```python
from build123d import *

# Parameters (mm, degrees)
TOP_PLATE_R             = 1
TOP_PLATE_R_2           = 2
TOP_PLATE_W             = 16.5
TOP_PLATE_H             = 8.5
TOP_PLATE_W_2           = 6
TOP_PLATE_H_2           = 18
TOP_PLATE_W_3           = 14
TOP_PLATE_H_3           = 12
TOP_PLATE_EXTRUDE_DEPTH = 2


with BuildPart() as part:
    # Top Plate → Top Plate Extrude (new body)
    with BuildSketch(Plane(origin=(0, 0, 0), x_dir=(1, 0, 0), z_dir=(0, 1, 0))):
        with BuildLine():
            Line((-38, 17.25), (-42.5, 17.25))
            Line((-42.5, 17.25), (-42.5, 14.926611549))
            Line((-42.5, 14.926611549), (-48, 14.926611549))
            Line((-48, 14.926611549), (-48, 10))
            Line((-48, 10), (-46.8, 10))
            ThreePointArc((-46.8, 10), (-46.587867966, 9.912132034), (-46.5, 9.7))
            Line((-46.5, 9.7), (-46.5, -9.7))
            ThreePointArc((-46.5, -9.7), (-46.587867966, -9.912132034), (-46.8, -10))
            Line((-46.8, -10), (-48, -10))
            Line((-48, -10), (-48, -14.926611549))
            Line((-48, -14.926611549), (-42.5, -14.926611549))
            Line((-42.5, -14.926611549), (-42.5, -17.25))
            Line((-42.5, -17.25), (-38, -17.25))
            Line((-38, -17.25), (-38, -14.926611549))
            Line((-38, -14.926611549), (-18, -14.926611549))
            Line((-18, -14.926611549), (-18, -17.25))
            Line((-18, -17.25), (-14, -17.25))
            Line((-14, -17.25), (-14, -14.926611549))
            Line((-14, -14.926611549), (6, -14.926611549))
            Line((6, -14.926611549), (6, -17.25))
            Line((6, -17.25), (10, -17.25))
            Line((10, -17.25), (10, -14.926611549))
            Line((10, -14.926611549), (34, -14.926611549))
            Line((34, -14.926611549), (34, -17.25))
            Line((34, -17.25), (47, -17.25))
            ThreePointArc((47, -17.25), (47.707106781, -16.957106781), (48, -16.25))
            Line((48, -16.25), (48, 16.25))
            ThreePointArc((48, 16.25), (47.707106781, 16.957106781), (47, 17.25))
            Line((47, 17.25), (34, 17.25))
            Line((34, 17.25), (34, 14.926611549))
            Line((34, 14.926611549), (10, 14.926611549))
            Line((10, 14.926611549), (10, 17.25))
            Line((10, 17.25), (6, 17.25))
            Line((6, 17.25), (6, 14.926611549))
            Line((6, 14.926611549), (-14, 14.926611549))
            Line((-14, 14.926611549), (-14, 17.25))
            Line((-14, 17.25), (-18, 17.25))
            Line((-18, 17.25), (-18, 14.926611549))
            Line((-18, 14.926611549), (-38, 14.926611549))
            Line((-38, 14.926611549), (-38, 17.25))
        make_face()
        with Locations(Location((-45.5, -11.5, 0), (0, 0, 270))):
            Circle(TOP_PLATE_R, mode=Mode.SUBTRACT)
        with Locations(Location((-41, -11.5, 0), (0, 0, 270))):
            Circle(TOP_PLATE_R, mode=Mode.SUBTRACT)
        with BuildLine():
            Line((-25, -10.5), (-13.5, -10.5))
            ThreePointArc((-13.5, -10.5), (-12.5, -11.5), (-13.5, -12.5))
            Line((-13.5, -12.5), (-25, -12.5))
            ThreePointArc((-25, -12.5), (-26, -11.5), (-25, -10.5))
        make_face(mode=Mode.SUBTRACT)
        with Locations(Location((44, -13.25, 0), (0, 0, 270))):
            Circle(TOP_PLATE_R_2, mode=Mode.SUBTRACT)
        with Locations((21.75, -6.75)):
            Rectangle(TOP_PLATE_W, TOP_PLATE_H, mode=Mode.SUBTRACT)
        with Locations((36, -0.25)):
            Rectangle(TOP_PLATE_W_2, TOP_PLATE_H_2, mode=Mode.SUBTRACT)
        with Locations((-31.5, 0)):
            Rectangle(TOP_PLATE_W_3, TOP_PLATE_H_3, mode=Mode.SUBTRACT)
        with Locations((-8.098292563, 0)):
            Rectangle(TOP_PLATE_W_3, TOP_PLATE_H_3, mode=Mode.SUBTRACT)
        with Locations(Location((-45.5, 11.5, 0), (0, 0, 270))):
            Circle(TOP_PLATE_R, mode=Mode.SUBTRACT)
        with Locations(Location((-41, 11.5, 0), (0, 0, 270))):
            Circle(TOP_PLATE_R, mode=Mode.SUBTRACT)
        with BuildLine():
            ThreePointArc((-13.5, 12.5), (-12.5, 11.5), (-13.5, 10.5))
            Line((-13.5, 10.5), (-25, 10.5))
            ThreePointArc((-25, 10.5), (-26, 11.5), (-25, 12.5))
            Line((-25, 12.5), (-13.5, 12.5))
        make_face(mode=Mode.SUBTRACT)
        Polygon((4.9, 9.249999917), (10.4, 9.249999917), (10.4, -8.75), (4.901707437, -8.750000002), align=None, mode=Mode.SUBTRACT)
        with Locations((21.75, 6.75)):
            Rectangle(TOP_PLATE_W, TOP_PLATE_H, mode=Mode.SUBTRACT)
        with BuildLine():
            ThreePointArc((42, 7.886262649), (43.5, 9.386262649), (45, 7.886262649))
            Line((45, 7.886262649), (45, -2.113737351))
            ThreePointArc((45, -2.113737351), (43.5, -3.613737351), (42, -2.113737351))
            Line((42, -2.113737351), (42, 7.886262649))
        make_face(mode=Mode.SUBTRACT)
        with Locations(Location((44, 12.75, 0), (0, 0, 270))):
            Circle(TOP_PLATE_R_2, mode=Mode.SUBTRACT)
    extrude(amount=TOP_PLATE_EXTRUDE_DEPTH)


solid = part.part
```
Verification items for the finished model (mm, model axes). A direction names the side the tool comes from. Round coordinates to 2 decimals unless told otherwise and drop trailing zeros. Order: outer loops, then holes, each group sorted by start corner. A loop starts at its lowest first (then second) coordinate and runs counter-clockwise, first axis right, second up. Notation, with made-up numbers: (77.5, 74) -> (106.5, 74) arc R6 ccw to (106.5, 82) -> close; hole circle Ø1 at (41, 33). An arc over 180 degrees is marked (long way). Put each result on its own line as item: value. Start each with the question number.
(1) Section check B-B (z = -1.5). Enter the section's corners in (x, y).
(2) Draft check along Z on faces 4 (the face through (-16, 1, -17.25)), 5 (the face through (43.467, 0.986, -9.386)), 6 (the face through (-40, 1, 17.25)). Enter one of: +Z half, -Z half, draft (parallel to the pull), parting line (faces both ways), or undercut.
(3) Tool access check on faces 1 (the face through (-18, 1, 16)), 2 (the face through (-4, 1, -14.927)), 3 (the face through (33, 1, 0)). Record the directions out of +Z, -Z, +X, -X, +Y, -Y that give a thin tool (end or side, any length) a straight path to the whole face; none if there is none.
(4) Section check C-C (x = 22). Enter the section's corners in (y, z), then the cut area to 3 significant figures.
(5) Section check A-A (x = 36). Enter the section's corners in (y, z), then the cut area to 3 significant figures.
(6) Material ranges on line 1 along X through (y, z) = (1.65, 4.5); line 2 along X through (y, z) = (0.2, -16); line 3 along X through (y, z) = (0.8, -7.5), recorded low to high.
(7) Depth check by flat-ended pin: pin 1 Ø2 at (x, z) = (-37, -4) entering from -Y; pin 2 Ø0.6 at (x, y) = (-4, 1.5) entering from +Z; pin 3 Ø0.6 at (x, y) = (-6.5, 1) entering from -Z. Enter the tip coordinate at first touch or a pass-through.
(8) Section check D-D (y = 1.1). State how many separate pieces and enclosed holes the cut face has, then the cut area to 3 significant figures.
Completed:
1. outline: (-46.5, 0) -> (-38.5, 0) -> (-38.5, 2) -> (-46.5, 2) -> close; (-24.5, 0) -> (-15.1, 0) -> (-15.1, 2) -> (-24.5, 2) -> close; (-1.1, 0) -> (4.9, 0) -> (4.9, 2) -> (-1.1, 2) -> close; (10.4, 0) -> (33, 0) -> (33, 2) -> (10.4, 2) -> close; (39, 0) -> (42, 0) -> (42, 2) -> (39, 2) -> close; (45, 0) -> (48, 0) -> (48, 2) -> (45, 2) -> close
2. face 4: -Z half
2. face 5: undercut
2. face 6: +Z half
3. face 1: +Z, +Y, -Y
3. face 2: -Z, +Y, -Y
3. face 3: +Y, -Y
4. outline: (0, -14.93) -> (2, -14.93) -> (2, -11) -> (0, -11) -> close; (0, -2.5) -> (2, -2.5) -> (2, 2.5) -> (0, 2.5) -> close; (0, 11) -> (2, 11) -> (2, 14.93) -> (0, 14.93) -> close
4. area: 25.7 mm2
5. outline: (0, -17.25) -> (2, -17.25) -> (2, -8.75) -> (0, -8.75) -> close; (0, 9.25) -> (2, 9.25) -> (2, 17.25) -> (0, 17.25) -> close
5. area: 33.0 mm2
6. line 1: x = -46.5 to -38.5, -24.5 to -15.1, -1.1 to 4.9, 10.4 to 13.5, 30 to 33, 39 to 48
6. line 2: x = -42.5 to -38, -18 to -14, 6 to 10, 34 to 48
6. line 3: x = -46.5 to 4.9, 10.4 to 13.5, 30 to 33, 39 to 42, 45 to 48
7. pin 1: passes through
7. pin 2: stops at z = 14.93
7. pin 3: stops at z = -14.93
8. separate pieces: 1
8. enclosed holes: 15
8. area: 2,010 mm2
